Job drawing, mm, ordinate dimensions from the low corner. One solid piece. Give positions to 0.01 mm unless a question says otherwise; leave off trailing zeros. Order: outer loops, then holes, each group sorted by start corner. A loop starts at its lowest first (then second) coordinate and runs counter-clockwise, first axis right, second up. Notation, with made-up numbers: M 6,-22.75 L 64,-22.75 A21 cw 64,14.25 Z; hole C 25,-28.75 d8. An arc over 180 degrees is marked long. One line per question, with ' | ' between items.
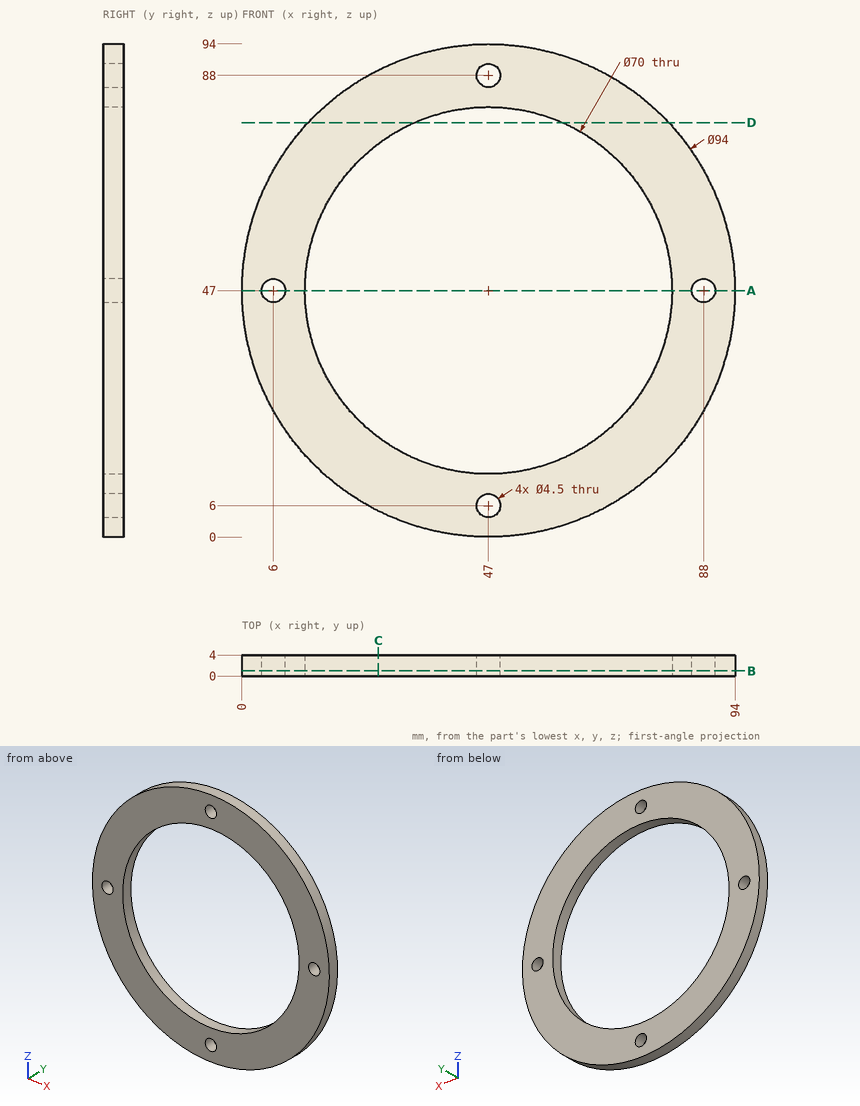
1. Probe L1, parallel to X at y = 1.2, z = 47; L2, parallel to Z at x = 60.5, y = 2; L3, parallel to Z at x = 70.5, y = 2.3. List the from-to ranges inside material, lowest first. Write a range as from..to.
Worked out:
L1: x = 0..3.75, 8.25..12, 82..85.75, 90.25..94 | L2: z = 1.98..14.71, 79.29..92.02 | L3: z = 6.3..21.06, 72.94..87.7
2. Slice it at D-D on z = 79. Give the cut face in (x, y), then the cut area to 3 significant figures.
Worked out:
outline: M 12.58,0 L 32.82,0 L 32.82,4 L 12.58,4 Z; M 61.18,0 L 81.42,0 L 81.42,4 L 61.18,4 Z | area: 162 mm2
3. Slice it at A-A on z = 47. Give the cut face in (x, y), then the cut area to 3 significant figures.
Worked out:
outline: M 0,0 L 3.75,0 L 3.75,4 L 0,4 Z; M 8.25,0 L 12,0 L 12,4 L 8.25,4 Z; M 82,0 L 85.75,0 L 85.75,4 L 82,4 Z; M 90.25,0 L 94,0 L 94,4 L 90.25,4 Z | area: 60.0 mm2
4. Slice it at B-B on y = 1. Give the cut face in (x, z), then the cut area to 3 significant figures.
Worked out:
outline: C 47,47 d94; hole C 6,47 d4.5; hole C 47,47 d70; hole C 47,6 d4.5; hole C 47,88 d4.5; hole C 88,47 d4.5 | area: 3,030 mm2
5. Drop flat-ended pins along their axis: pin 1 (8 mm diameter, centred on x = 73, z = 39, fed in from +Y); pin 2 (7 mm diameter, centred on x = 88, z = 47, fed in from -Y); pin 3 (2 mm diameter, centred on y = 1, z = 47, fed in from +X). Give the stop position or say it passes through.
Worked out:
pin 1: passes through | pin 2: stops at y = 0 | pin 3: stops at x = 94
6. Slice it at C-C on x = 26. Give the cut face in (y, z), then the cut area to 3 significant figures.
Worked out:
outline: M 0,4.95 L 4,4.95 L 4,19 L 0,19 Z; M 0,75 L 4,75 L 4,89.05 L 0,89.05 Z | area: 112 mm2
